Work out the finished part from the listing and answer in its coordinate system (mm). Face numbers are marked on the shaded views. A direction names the side the tool comes from. Give positions to 0.01 mm unless a question says otherwise; leave off trailing zeros. Loops run counter-clockwise (first coordinate to the right, second up) from the corner with the lowest first, then second, coordinate; pieces in that order, holes last. Notation, with made-up numbers: (-38, -28.75) - (-14, -28.75) arc R33 ccw to (-14, 9.25) - close; hole circle Ø2 at (-37, 64). An arc over 180 degrees is marked (long way). One line per question, with ' | ' between items. Start each with the question number.
1. Section D-D (y = 7.25) is taken. Determine the outline of the cut face in (x, z), plus the area to 3 significant figures.
2. Which of the six approach directions +Z, -Z, +X, -X, +Y, -Y give full straight-line access (tool end or side, diameter ignored) to the marked faces 1 and 2?
3. Each of these flat-tipped pins is pushed along its axis until it touches: pin 1 (4 mm diameter, centred on x = 7, y = 2, fed in from -Z); pin 2 (2 mm diameter, centred on y = 7.5, z = 4.5, fed in from +X); pin 3 (6 mm diameter, centred on x = 8.5, y = 5, fed in from -Z). Where does it stop, or does it pass through?
4. Section A-A (y = 0) is taken. Determine the outline of the cut face in (x, z).
5. Section C-C (z = 5.75) is taken. Determine the outline of the cut face in (x, y), plus the area to 3 significant figures.
6. Find the intervals of material crossed by line 1 (Z direction, x = 1.5, y = -7.75); line 2 (Z direction, x = 4, y = -3.5); line 3 (X direction, y = 8.5, z = 6.25), in increasing order.
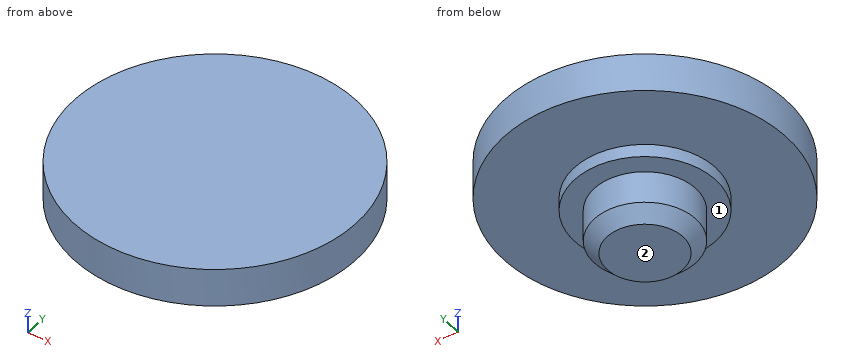
from build123d import *

# Parameters (mm, degrees)
F2_SIZE = 1


with BuildPart() as f1:
    # F0 (on Front) → F1 (revolve)
    with BuildSketch(Plane.XZ):
        Polygon((-3.95, 0), (0, 0), (0, 7.5), (-11, 7.5), (-11, 4.5), (-5.5, 4.5), (-5.5, 3.5), (-3.95, 3.5), align=None)
    revolve(axis=Axis((0, 0, 3.75), (0, 0, 1)))

    # F2
    f2_edges = [f1.edges().sort_by_distance(p)[0] for p in [
        (3.95, 0, 0),
    ]]
    chamfer(f2_edges, length=F2_SIZE)


solid = f1.part
Conclusion:
1) outline: (-8.27, 4.5) - (8.27, 4.5) - (8.27, 7.5) - (-8.27, 7.5) - close | area: 49.6 mm²
2) face 1: -Z | face 2: -Z, +X, -X, +Y, -Y
3) pin 1: z = 3.5 | pin 2: x = 8.87 | pin 3: z = 4.5
4) outline: (-11, 4.5) - (-5.5, 4.5) - (-5.5, 3.5) - (-3.95, 3.5) - (-3.95, 1) - (-2.95, 0) - (2.95, 0) - (3.95, 1) - (3.95, 3.5) - (5.5, 3.5) - (5.5, 4.5) - (11, 4.5) - (11, 7.5) - (-11, 7.5) - close
5) outline: circle Ø22 at (0, 0) | area: 380 mm²
6) line 1: 4.5 to 7.5 | line 2: 3.5 to 7.5 | line 3: -6.98 to 6.98
